Input: part model. Units: mm. Frame: model coordinates. A direction names the side the tool comes from. Round coordinates to 2 decimals unless told otherwise and drop trailing zeros. Loops run counter-clockwise (first coordinate to the right, second up) from the corner with the lowest first, then second, coordinate; pieces in that order, holes last. Notation, with made-up numbers: (-27, 50.25) -> (-12, 50.25) arc R16 cw to (-12, 61.25) -> close; hole circle Ø11 at (32, -28.75). An arc over 180 degrees is marked (long way). Answer as a JSON object with one key per item and string values.
```python
from build123d import *

# Parameters (mm, degrees)
F2_R    = 0.5
F3_SIZE = 1
F4_SIZE = 0.5
F5_R    = 0.75


with BuildPart() as f1:
    # F0 (on Right) → F1 (revolve)
    with BuildSketch(Plane.YZ):
        with BuildLine():
            Line((19.5, 3), (18.25, 3))
            Line((18.25, 3), (18.25, 1.64))
            ThreePointArc((18.25, 1.64), (19.89, 0), (18.25, -1.64))
            Line((18.25, -1.64), (18.25, -3))
            Line((18.25, -3), (23.25, -3))
            Line((23.25, -3), (23.25, 0))
            Line((23.25, 0), (21.5, 0))
            Line((21.5, 0), (21.5, 3))
            Line((21.5, 3), (19.5, 3))
        make_face()
        Polygon((19.5, 11), (19.5, 3), (21.5, 3), (21.5, 13), (19.5, 13), align=None)
    revolve(axis=Axis((0, 0, 4.880332), (0, 0, 1)))

    # F2
    f2_edges = [f1.edges().sort_by_distance(p)[0] for p in [
        (0, -21.5, 0),
    ]]
    fillet(f2_edges, radius=F2_R)

    # F3
    f3_edges = [f1.edges().sort_by_distance(p)[0] for p in [
        (0, -23.25, -3),
    ]]
    chamfer(f3_edges, length=F3_SIZE)

    # F4
    f4_edges = [f1.edges().sort_by_distance(p)[0] for p in [
        (0, -21.5, 13),
        (0, -19.5, 13),
    ]]
    chamfer(f4_edges, length=F4_SIZE)

    # F5
    f5_edges = [f1.edges().sort_by_distance(p)[0] for p in [
        (0, -19.5, 3),
    ]]
    fillet(f5_edges, radius=F5_R)


solid = f1.part
```
1) Reachability of faces 1 (the face through (17.816, -3.956, 2.31)), 2 (the face through (9, 21, 0)) from +Z, -Z, +X, -X, +Y, -Y: full face, straight path, thin tool, end or side. Return the list, or none.
Output:
{"face 1": "+Z, -Z", "face 2": "+Z"}
2) Contact query for flat-ended pins moving along their axis: P1, Ø4, axis at y = 11.5, z = 0.5, coming from the -X side; P2, Ø1, axis at x = 6.5, z = 1, coming from the -Y side; P3, Ø6, axis at y = -17.5, z = 7, coming from the -X side. Output: stop coordinate, or through.
Output:
{"P1": "stops at x = -21.19", "P2": "stops at y = -20.65", "P3": "stops at x = -15.87"}
3) Section C-C, the plane z = 5.75. Output: boundary loops of the cut face in (x, y).
Output:
{"outline": "circle Ø43 at (0, 0); hole circle Ø39 at (0, 0)"}
4) Ray query, probe 1 along Y at (x, z) = (0, -2); probe 2 along X at (y, z) = (0, 2.2); probe 3 along Y at (x, z) = (0, 8). Return the intervals inside material, ascending.
Output:
{"probe 1": "y = -23.25 to -18.25, 18.25 to 23.25", "probe 2": "x = -21.5 to -18.25, 18.25 to 21.5", "probe 3": "y = -21.5 to -19.5, 19.5 to 21.5"}
5) Draft query along X for faces 3 (the face through (-18.2, 3.4, -3)), 4 (the face through (-21.317, -2.799, 6.584)), 5 (the face through (18, 4, 3)). Return one class per face: +X half, -X half, draft (parallel to the pull), parting line (faces both ways), or undercut.
Output:
{"face 3": "draft", "face 4": "parting line", "face 5": "undercut"}
